The model under review builds one solid part; all positions refer to its coordinate system, in mm. Face numbers are marked on the shaded views. Coordinates: 2 decimals unless noted, no trailing zeros. Write each loop counter-clockwise with the first axis right and the second up, starting at its lowest first coordinate (ties: lowest second). Pieces come first, ordered by that corner, then holes. Notation, with made-up numbers: (49.5, 61.5) - (57.5, 61.5) arc R33 cw to (57.5, 92.5) - close; hole circle Ø7 at (5, -20.75). An arc over 180 degrees is marked (long way). Put each result on its own line as item: value. Start each with the question number.
Item 1: Consider section A-A on x = 0. Give the boundary of the cut face in (y, z), then the cut area to 3 significant figures.
Item 2: To check wall thickness, follow L1, parallel to Y at x = 36.5, z = -1.5; L2, parallel to Y at x = 23.5, z = -7.5; L3, parallel to Z at x = -22.5, y = 73.5. State the ranges of each line that lie inside material, in increasing order. Write a range as [from, to].
Item 3: Consider section C-C on z = 18.5. Give the boundary of the cut face in (x, y) (3 decimals), then the cut area to 3 significant figures.
Item 4: Consider section B-B on y = 69. Give the boundary of the cut face in (x, z) (3 decimals), then the cut area to 3 significant figures.
Item 5: Mouldability with a two-part tool opening along X and no side actions: class the marked faces 1, 2, 3 and 4 as pulls with the +X half, pulls with the -X half, needs draft (parallel to the pull), parting line crosses it, or undercut.
Item 6: For pin 1 (3 mm diameter, centred on y = 12.702, z = 34.925, fed in from +X) (3 decimals); pin 2 (3 mm diameter, centred on y = 12.702, z = -34.925, fed in from -X) (3 decimals); pin 3 (1.5 mm diameter, centred on x = 24.5, z = -21, fed in from +Y), all flat-tipped, find the tip position at first contact; note any pin that passes through.
Item 7: Consider section D-D on y = 47.5. Give the boundary of the cut face in (x, z) (3 decimals).
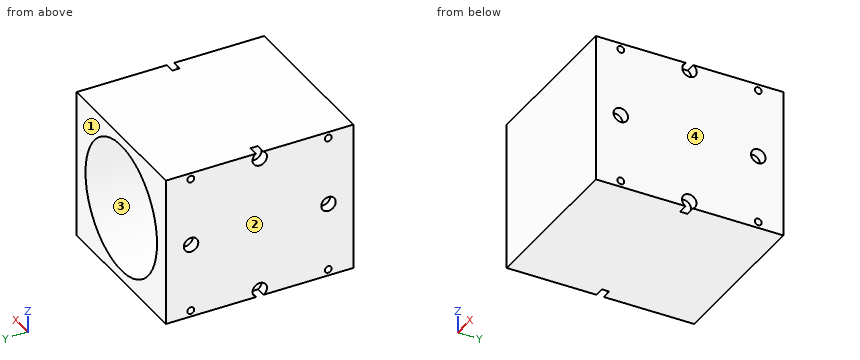
Autodesk Inventor part; units mm, degrees
ref_plane "YZ Plane" through (0, 0, 0) normal (1, 0, 0) x (0, 1, 0)
ref_plane "XZ Plane" through (0, 0, 0) normal (0, 1, 0) x (-1, 0, 0)
ref_plane "XY Plane" through (0, 0, 0) normal (0, 0, 1) x (1, 0, 0)
sketch "Sketch1" plane through (0, 0, 0) normal (0, 1, 0) x (-1, 0, 0)
  line L0 (41.275, -38.1) -> (-41.275, -38.1)
  line L1 (-41.275, -38.1) -> (-41.275, 38.1)
  line L2 (-41.275, 38.1) -> (41.275, 38.1)
  line L3 (41.275, 38.1) -> (41.275, -38.1)
  circle A0 centre (0, 0) radius 4.5409
  dimension "d3" = 82.55
  dimension "d4" = 76.2
extrude "block" add sketch "Sketch1" along normal blind 95.25 contours L0 L1 L2 L3 | A0
sketch "Sketch2" plane through (0, 95.25, 0) normal (0, 1, 0) x (1, 0, 0)
  circle A0 centre (0, 0) radius 33.147
  dimension "d7" = 66.294
extrude "hole" cut sketch "Sketch2" against normal blind 88.9
sketch "Sketch4" plane through (41.275, 0, 38.1) normal (1, 0, 0) x (0, 0, -1)
  line L0 (76.2, 85.6) -> (76.2, 9.4)
  line L1 (0, 9.4) -> (0, 85.6)
  line L2 (38.227, 85.727) -> (38.102, 85.727)
  line L3 (0, 0) -> (0, 95.25)
  line L4 (0, 47.625) -> (0, 47.375)
  line L5 (76.2, 0) -> (76.2, 95.25)
  line L6 (76.2, 47.625) -> (76.2, 47.5)
  line L7 (8.3242, 59.8735) -> (8.4492, 59.8735)
  line L8 (38.102, 85.727) -> (38.102, 82.552)
  circle A0 centre (38.102, 82.552) radius 3.683
  circle A1 centre (3.175, 47.625) radius 3.683
  circle A2 centre (38.102, 12.702) radius 3.683
  circle A3 centre (73.025, 47.5) radius 3.683
  line L9 (0, 47.625) -> (3.175, 47.625)
  line L10 (38.102, 82.425) -> (38.102, -13.1059)
  line L11 (3.175, 47.625) -> (115.5999, 47.625)
  circle A4 centre (73.025, 47.625) radius 0.0045
  point P0 (38.1, 0)
  dimension "d10" = 76.2
  dimension "d11" = 76.2
  dimension "d21" = 3.175
  dimension "d30" = 7.366
  dimension "d32" = 7.366
  dimension "d33" = 7.366
  dimension "d34" = 7.366
  dimension "d35" = 3.175
extrude "Extrusion3" cut sketch "Sketch4" against normal blind 5.08
sketch "Sketch5" plane through (-41.275, 0, -38.1) normal (-1, 0, 0) x (0, 0, 1)
  line L0 (0, 85.6) -> (76.2, 85.6)
  line L1 (76.2, 85.6) -> (76.2, 9.4)
  line L2 (76.2, 9.4) -> (0, 9.4)
  line L3 (0, 9.4) -> (0, 85.6)
  line L4 (38.1, 85.6) -> (37.975, 85.6)
  line L5 (38.1, 9.4) -> (38.225, 9.4)
  line L6 (0, 0) -> (0, 95)
  line L7 (0, 47.5) -> (0, 47.375)
  line L8 (76.2, 0) -> (76.2, 95)
  line L9 (76.2, 47.5) -> (76.2, 47.375)
  line L10 (8.3242, 59.8735) -> (8.4492, 59.8735)
  line L11 (0, 47.375) -> (3.175, 47.375)
  line L12 (37.975, 85.6) -> (37.975, 82.425)
  line L13 (76.2, 47.375) -> (73.025, 47.375)
  line L14 (38.225, 9.4) -> (38.225, 12.575)
  circle A0 centre (3.175, 82.552) radius 1.7526
  circle A1 centre (73.025, 12.702) radius 1.7526
  circle A2 centre (3.175, 12.702) radius 1.7526
  circle A3 centre (73.025, 82.552) radius 1.7526
  point P0 (38.1, 0)
  point P1 (38.1, 0)
  dimension "d24" = 76.2
  dimension "d25" = 76.2
  dimension "d26" = 3.175
  dimension "d27" = 3.175
  dimension "d28" = 3.175
  dimension "d29" = 3.175
  dimension "d38" = 3.5052
  dimension "d39" = 3.5052
  dimension "d40" = 3.5052
  dimension "d41" = 3.5052
extrude "Extrusion4" cut sketch "Sketch5" against normal blind 11.43 contours A0 | A1 | A2 | A3
sketch "Sketch6" plane through (-41.275, 0, -38.1) normal (-1, 0, 0) x (0, 0, 1)
  circle A0 centre (38.098, 82.425) radius 3.683
  circle A1 centre (38.098, 82.425) radius 3.683
  circle A2 centre (3.175, 47.5) radius 3.683
  circle A3 centre (37.973, 12.575) radius 3.683
  circle A4 centre (37.973, 12.575) radius 3.683
  arc A5 (76.2, 49.3763) -> (76.2, 45.6433) centre (73.025, 47.5098) ccw
  circle A6 centre (73.025, 47.5098) radius 3.683
  line L0 (76.2, 95.0156) -> (0, 95.0156)
  line L1 (0, 0.0156) -> (0, 45.6334)
  line L2 (76.2, 0.0156) -> (76.2, 95.0156)
  line L3 (4.85, 95) -> (71.35, 95)
  line L4 (0, 0.0156) -> (76.2, 0.0156)
  arc A7 (0, 45.6334) -> (0, 49.3666) centre (3.175, 47.5) ccw
  point P0 (38.1, 0)
  point P1 (0, 95.0156)
extrude "Extrusion5" cut sketch "Sketch6" against normal blind 5.08
sketch "Sketch9" plane through (41.275, 0, 38.1) normal (1, 0, 0) x (0, 0, -1)
  circle A0 centre (3.175, 82.552) radius 1.7526
  circle A1 centre (3.175, 82.552) radius 1.7526
  circle A2 centre (3.175, 12.702) radius 1.7526
  circle A3 centre (3.175, 12.702) radius 1.7526
  circle A4 centre (73.025, 12.702) radius 1.7526
  circle A5 centre (73.025, 12.702) radius 1.7526
  circle A6 centre (73.025, 82.552) radius 1.7526
  circle A7 centre (73.025, 82.552) radius 1.7526
  point P0 (38.1, 0)
extrude "Extrusion6" cut sketch "Sketch9" against normal blind 11.43
properties part number "mid_block"
Report:
1. outline: (0, -38.1) - (95.25, -38.1) - (95.25, -33.15) - (6.35, -33.15) - (6.35, 33.15) - (95.25, 33.15) - (95.25, 38.1) - (0, 38.1) - close
1. area: 1,360 mm²
2. L1: [0, 9.34], [16.07, 79.19], [85.92, 95.25]
2. L2: [0, 6.35]
2. L3: [-38.1, -24.34], [24.34, 38.1]
3. outline: (-41.275, 0) - (41.275, 0) - (41.275, 95.25) - (27.504, 95.25) - (27.504, 6.35) - (-27.504, 6.35) - (-27.504, 95.25) - (-41.275, 95.25) - close
3. area: 2,970 mm²
4. outline: (-41.275, -38.1) - (41.275, -38.1) - (41.275, 38.1) - (-41.275, 38.1) - close; hole circle Ø66.294 at (0, 0)
4. area: 2,840 mm²
5. face 1: needs draft
5. face 2: pulls with the -X half
5. face 3: undercut
5. face 4: pulls with the +X half
6. pin 1: x = 29.845
6. pin 2: x = -29.845
6. pin 3: y = 6.35
7. outline: (-41.275, -31.242) - (-36.195, -31.242) - (-36.195, -38.1) - (36.195, -38.1) - (36.195, -31.242) - (41.275, -31.242) - (41.275, 31.244) - (36.195, 31.244) - (36.195, 38.1) - (-36.195, 38.1) - (-36.195, 31.242) - (-41.275, 31.242) - close; hole circle Ø66.294 at (0, 0)
